```python
from build123d import *

# Parameters (mm, degrees)
SKETCH1_W           = 46
SKETCH1_H           = 79
BOSS_EXTRUDE1_DEPTH = 2
SKETCH2_W           = 2
SKETCH2_H           = 5
BOSS_EXTRUDE2_DEPTH = 3
BOSS_EXTRUDE3_DEPTH = 5
FILLET1_R           = 0.6
SKETCH4_W           = 46
SKETCH4_H           = 79
SKETCH4_W_2         = 42
SKETCH4_H_2         = 75
CUT_EXTRUDE1_DEPTH  = 10
SKETCH5_W           = 42
SKETCH5_H           = 1
BOSS_EXTRUDE4_DEPTH = 2
SKETCH6_W           = 42
SKETCH6_H           = 1
BOSS_EXTRUDE5_DEPTH = 2
FILLET2_R           = 1
SKETCH7_W           = 5.220052767
SKETCH7_H           = 2.493732105
SKETCH7_W_2         = 4.447072359
SKETCH7_H_2         = 2.905988322
CUT_EXTRUDE2_DEPTH  = 10
BOSS_EXTRUDE6_DEPTH = 5
FILLET3_R           = 0.6


with BuildPart() as part:
    # Sketch1 → Boss-Extrude1 (new body)
    with BuildSketch(Plane.XY):
        with Locations((23, -39.5)):
            Rectangle(SKETCH1_W, SKETCH1_H)
    extrude(amount=BOSS_EXTRUDE1_DEPTH)

    # Sketch2 → Boss-Extrude2 (add)
    with BuildSketch(Plane.XY.offset(2)):
        with Locations((3, -38.5)):
            Rectangle(SKETCH2_W, SKETCH2_H)
        with Locations((43, -38.5)):
            Rectangle(SKETCH2_W, SKETCH2_H)
    extrude(amount=BOSS_EXTRUDE2_DEPTH)

    # Sketch3 → Boss-Extrude3 (add)
    with BuildSketch(Plane.XZ.offset(41)):
        Polygon((2, 7), (0, 5), (2, 5), (4, 5), (4, 7), align=None)
        Polygon((44, 7), (42, 7), (42, 5), (46, 5), align=None)
    extrude(amount=-BOSS_EXTRUDE3_DEPTH)

    # Fillet1
    fillet1_edges = [part.edges().sort_by_distance(p)[0] for p in [
        (0, -38.5, 5),
        (46, -38.5, 5),
    ]]
    fillet(fillet1_edges, radius=FILLET1_R)

    # Sketch4 → Cut-Extrude1 (cut)
    with BuildSketch(Plane.XY.offset(2)):
        with Locations((23, -39.5)):
            Rectangle(SKETCH4_W, SKETCH4_H)
        with Locations((23, -39.5)):
            Rectangle(SKETCH4_W_2, SKETCH4_H_2, mode=Mode.SUBTRACT)
    extrude(amount=-CUT_EXTRUDE1_DEPTH, mode=Mode.SUBTRACT)

    # Sketch5 → Boss-Extrude4 (add)
    with BuildSketch(Plane.XY.offset(2)):
        with Locations((23, -1.5)):
            Rectangle(SKETCH5_W, SKETCH5_H)
    extrude(amount=-BOSS_EXTRUDE4_DEPTH)

    # Sketch6 → Boss-Extrude5 (add)
    with BuildSketch(Plane.XY.offset(2)):
        with Locations((23, -0.5)):
            Rectangle(SKETCH6_W, SKETCH6_H)
    extrude(amount=-BOSS_EXTRUDE5_DEPTH)

    # Fillet2
    fillet2_edges = [part.edges().sort_by_distance(p)[0] for p in [
        (44, -77, 1),
        (2, -77, 1),
    ]]
    fillet(fillet2_edges, radius=FILLET2_R)

    # Sketch7 → Cut-Extrude2 (cut)
    with BuildSketch(Plane.XZ.offset(41)):
        with Locations((1.389973616, 6.246866052)):
            Rectangle(SKETCH7_W, SKETCH7_H)
        with Locations((44.22353618, 6.452994161)):
            Rectangle(SKETCH7_W_2, SKETCH7_H_2)
    extrude(amount=-CUT_EXTRUDE2_DEPTH, mode=Mode.SUBTRACT)

    # Sketch8 → Boss-Extrude6 (add)
    with BuildSketch(Plane.XZ.offset(41)):
        Polygon((2, 5), (0, 2.5), (4, 2.5), (4, 5), align=None)
        Polygon((42, 2.5), (46, 2.5), (44, 5), (42, 5), align=None)
    extrude(amount=-BOSS_EXTRUDE6_DEPTH)

    # Fillet3
    fillet3_edges = [part.edges().sort_by_distance(p)[0] for p in [
        (0, -38.5, 2.5),
        (46, -38.5, 2.5),
    ]]
    fillet(fillet3_edges, radius=FILLET3_R)


solid = part.part
```
Part model, mm, in its own coordinate system. A direction names the side the tool comes from. Give positions to 0.01 mm unless a question says otherwise; leave off trailing zeros. Order: outer loops, then holes, each group sorted by start corner. A loop starts at its lowest first (then second) coordinate and runs counter-clockwise, first axis right, second up. Notation, with made-up numbers: (83, 1) - (109, 1) arc R22 cw to (109, 29) - close; hole circle Ø5 at (47.5, 76). An arc over 180 degrees is marked (long way). Use one line per item in the form item = value.
Item 1: Which spindle directions (+Z, -Z, +X, -X, +Y, -Y) get a long thin tool onto all of the face, cutting with end or side? Do faces 1 (the face through (3, -41, 4)), 2 (the face through (43, -36, 3)), 3 (the face through (42, -39, 3)), 4 (the face through (44, -39, 1)), 5 (the face through (2, -39, 1)). Say none if no direction does.
Solution:
face_1 = +Z, +X, -X, -Y
face_2 = +Z, +X, -X, +Y
face_3 = +Z, +Y, -Y
face_4 = -Z, +X, +Y, -Y
face_5 = -Z, -X, +Y, -Y
Item 2: Probe probe 1 along X at (y, z) = (-39, 3.05); probe 2 along Y at (x, z) = (43, 3.15); probe 3 along X at (y, z) = (-30, 1.75). List the from-to ranges inside material, lowest first. Write a range as from..to.
Solution:
probe_1 = 0.65..4, 42..45.35
probe_2 = -41..-36
probe_3 = 2..44
Item 3: Slice it at C-C on x = 20.5. Give the cut face in (y, z).
Solution:
outline = (-77, 0) - (0, 0) - (0, 2) - (-77, 2) - close
Item 4: Slice it at B-B on z = 1.15. Give the cut face in (x, y), and give its area (3 significant figures).
Solution:
outline = (2, -76) arc R1 ccw to (3, -77) - (43, -77) arc R1 ccw to (44, -76) - (44, 0) - (2, 0) - close
area = 3,230 mm2
Item 5: Slice it at A-A on y = -39. Give the cut face in (x, z).
Solution:
outline = (0.78, 3.47) arc R0.6 ccw to (1.25, 2.5) - (2, 2.5) - (2, 0) - (44, 0) - (44, 2.5) - (44.75, 2.5) arc R0.6 ccw to (45.22, 3.47) - (44, 5) - (42, 5) - (42, 2) - (4, 2) - (4, 5) - (2, 5) - close
Item 6: Slice it at D-D on y = -31. Give the cut face in (x, z).
Solution:
outline = (2, 0) - (44, 0) - (44, 2) - (2, 2) - close
Item 7: Pin check, flat tips, straight feed: pin 1 Ø6 at (x, y) = (8, -18.5) entering from +Z; pin 2 Ø2 at (y, z) = (-45.5, 1.5) entering from -X; pin 3 Ø1 at (x, z) = (31.5, 3) entering from -Y; pin 4 Ø1.5 at (x, z) = (44, 3) entering from -Y. Stop position of each tip, or through.
Solution:
pin_1 = 2
pin_2 = 2
pin_3 = through
pin_4 = -41
Item 8: Two-plate mould, pull along X, no slides. Class faces 6 (the face through (1.4, -38.53, 4.25)), 7 (the face through (4, -39, 3)), 8 (the face through (23, -38, 0)): released by +X, released by -X, zero draft, split by the parting line, or undercut.
Solution:
face_6 = released by -X
face_7 = undercut
face_8 = zero draft
